Read the model definition and answer for the solid it produces. Units are mm, in the model's axes. Face numbers are marked on the shaded views. Give positions to 0.01 mm unless a question says otherwise; leave off trailing zeros. Order: outer loops, then holes, each group sorted by start corner. A loop starts at its lowest first (then second) coordinate and runs counter-clockwise, first axis right, second up. Notation, with made-up numbers: (-29.5, -11) -> (17.5, -11) arc R23 cw to (17.5, 25) -> close; hole circle Ø4 at (-34.75, 17.5). An arc over 180 degrees is marked (long way). Answer as CSV lines item,"result". Start each with the question number.
1) The mould has two halves that part along X. Classify the marked faces 1, 2, 3 and 4: +X half, -X half, draft (parallel to the pull), parting line (faces both ways), or undercut.
2) Find section C-C (z = 0.4). Determine the outline of the cut face in (x, y).
3) Straight lines are drawn through the part: L1, parallel to X at y = 9.75, z = 3.4; L2, parallel to X at y = 10, z = 1.35; L3, parallel to X at y = 4.25, z = 1.7. For each, find the intervals that lie inside material, in ascending order. Write a range as from..to.
```python
from build123d import *

# Parameters (mm, degrees)
F0_W        = 14
F0_H        = 17.5
F1_DEPTH    = 3.7
F3_DEPTH    = 5.4
F4_R        = 3.69999
F5_R        = 3
F6_T1_DEPTH = 17.30001


# Not quite as in the source:
# - a fillet or chamfer that OpenCascade refuses, or shapes differently, is made with other operations: its cross-section is extruded or revolved along the edge and cut away or added
# - a fillet or chamfer is up to 0.001 mm smaller than in the source, because OpenCascade refuses the exact size


with BuildPart() as f1:
    # F0 (on Top) → F1 (new body)
    with BuildSketch(Plane.XY):
        with Locations((-0.4103374667, 3.4223956802)):
            Rectangle(F0_W, F0_H)
    extrude(amount=F1_DEPTH)

    # F2 (on face) → F3 (cut)
    with BuildSketch(Plane.XY.offset(3.7)):
        with BuildLine():
            Line((-5.3451164257, 9.1307080224), (-5.3451164257, 9.2324278445))
            ThreePointArc((-5.3451164257, 9.2324278445), (-5.3456139214, 9.1815679334), (-5.3451164257, 9.1307080224))
        make_face()
        with BuildLine():
            Line((-5.3451164257, 12.1723956802), (-5.3451164257, 9.2324278445))
            Line((-5.3451164257, 9.2324278445), (-5.3451164257, 9.1307080224))
            ThreePointArc((-5.3451164257, 9.1307080224), (-2.7588797704, 6.5816017765), (-0.1467657558, 9.1041843944))
            Line((-0.1467657558, 9.1041843944), (-0.055406418, 12.1723956802))
            Line((-0.055406418, 12.1723956802), (-5.3451164257, 12.1723956802))
        make_face()
    extrude(amount=-F3_DEPTH, mode=Mode.SUBTRACT)

    # F4 (radius 3.7 in the source; OpenCascade refuses exactly that, so slightly less here)
    f4_edges = [f1.edges().sort_by_distance(p)[0] for p in [
        (6.589663, 3.422396, 3.7),
    ]]
    fillet(f4_edges, radius=F4_R)

    # F5
    f5_edges = [f1.edges().sort_by_distance(p)[0] for p in [
        (-7.410337, -5.327604, 1.85),
    ]]
    fillet(f5_edges, radius=F5_R)

    # F6: fillet of radius 2 on 1 edges, made by hand

    # F6_s2 → F6_t1 (cut)
    with BuildSketch(Plane.YZ.offset(-9.4103374667)):
        with BuildLine():
            add(Edge.make_bspline(
                [(-5.3276043198, 1.7), (-5.3276043198, 3.7), (-3.3276043198, 3.7)],
                knots=[0, 0, 0, 1, 1, 1], degree=2, weights=[1, 1, 1]))
            Line((-3.3276043198, 3.7), (-5.3276043198, 3.7))
            Line((-5.3276043198, 3.7), (-5.3276043198, 1.7))
        make_face()
    extrude(amount=F6_T1_DEPTH, mode=Mode.SUBTRACT)


solid = f1.part
```
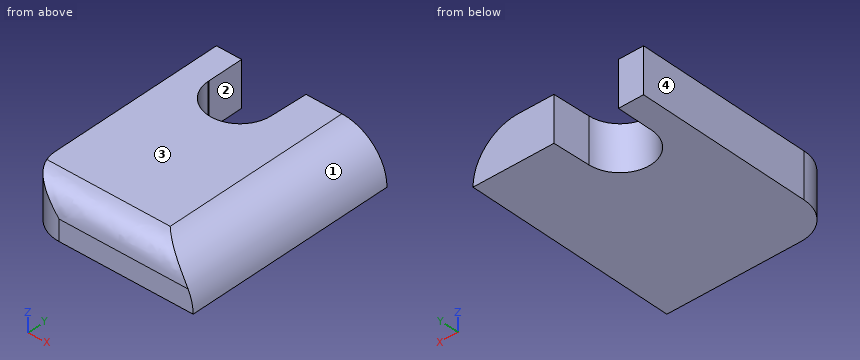
Findings below:
1,face 1,"+X half"
1,face 2,"undercut"
1,face 3,"draft"
1,face 4,"-X half"
2,outline,"(-7.41, -2.33) arc R3 ccw to (-4.41, -5.33) -> (6.57, -5.33) -> (6.57, 12.17) -> (-0.06, 12.17) -> (-0.15, 9.1) arc R2.6 cw to (-5.35, 9.23) -> (-5.35, 12.17) -> (-7.41, 12.17) -> close"
3,L1,"-7.41..-5.35, -0.13..4.35"
3,L2,"-7.41..-5.35, -0.12..6.33"
3,L3,"-7.41..6.18"
